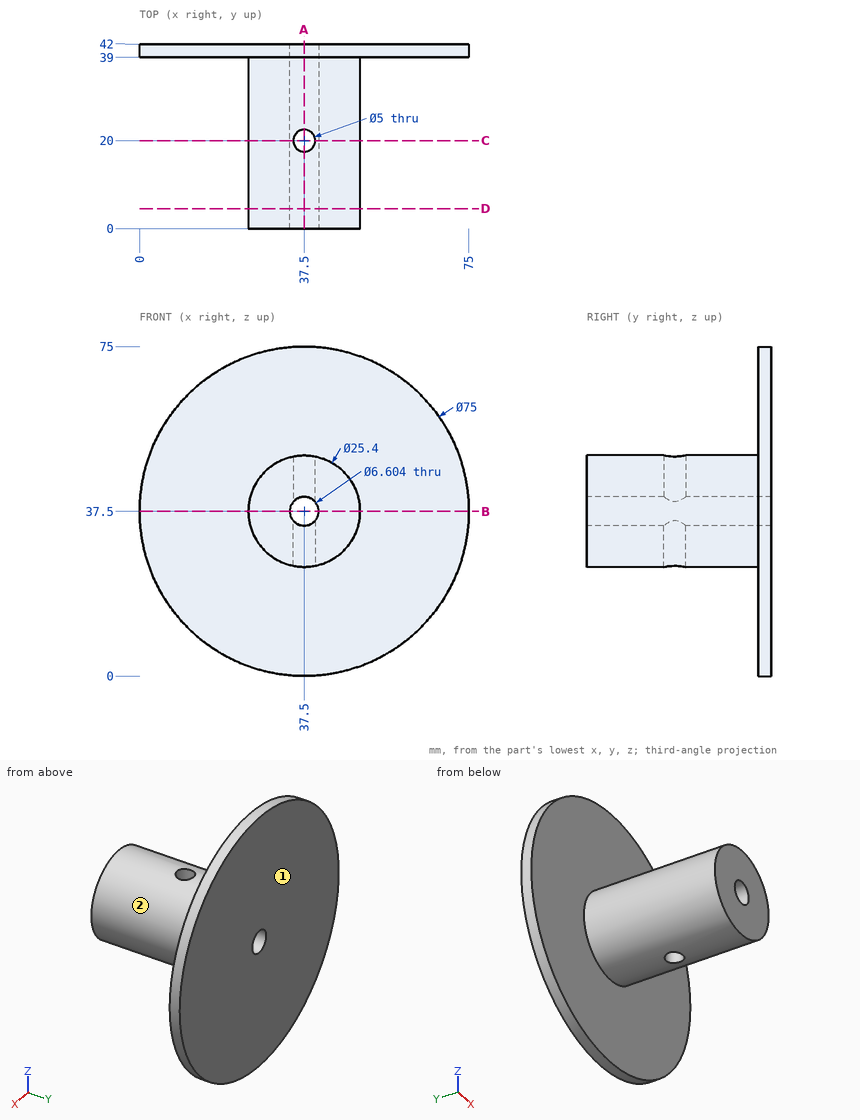
The figure shows three views and two pictorial views of one solid part (mm, origin at its lowest corner). Answer the questions. A direction names the side the tool comes from. Round coordinates to 2 decimals unless told otherwise and drop trailing zeros. Order: outer loops, then holes, each group sorted by start corner. A loop starts at its lowest first (then second) coordinate and runs counter-clockwise, first axis right, second up. Notation, with made-up numbers: (75, 75.5) -> (99, 75.5) arc R34 ccw to (99, 106.5) -> close; hole circle Ø2 at (22.5, -15). An arc over 180 degrees is marked (long way). Put each result on its own line as item: value.
Q1. Section D-D, the plane y = 4.5 is taken. Write down the section's boundary in (x, z), and give its area (3 significant figures).
Results list:
outline: circle Ø25.4 at (37.5, 37.5); hole circle Ø6.6 at (37.5, 37.5)
area: 472 mm^2
Q2. Section C-C, the plane y = 20 is taken. Write down the section's boundary in (x, z), and give its area (3 significant figures).
Results list:
outline: (35, 25.05) -> (35, 35.34) arc R3.3 cw to (35, 39.66) -> (35, 49.95) arc R12.7 ccw to start; (40, 25.05) arc R12.7 ccw to (40, 49.95) -> (40, 39.66) arc R3.3 cw to (40, 35.34) -> close
area: 376 mm^2
Q3. Section A-A, the plane x = 37.5 is taken. Write down the section's boundary in (y, z).
Results list:
outline: (0, 24.8) -> (17.5, 24.8) -> (17.5, 34.2) -> (0, 34.2) -> close; (0, 40.8) -> (17.5, 40.8) -> (17.5, 50.2) -> (0, 50.2) -> close; (22.5, 24.8) -> (39, 24.8) -> (39, 0) -> (42, 0) -> (42, 34.2) -> (22.5, 34.2) -> close; (22.5, 40.8) -> (42, 40.8) -> (42, 75) -> (39, 75) -> (39, 50.2) -> (22.5, 50.2) -> close
Q4. Which of the six approach directions +Z, -Z, +X, -X, +Y, -Y give full straight-line access (tool end or side, diameter ignored) to the marked faces 1 and 2?
Results list:
face 1: +Z, -Z, +X, -X, +Y
face 2: -Y
Q5. Consider line 1 along Z through (x, y) = (37.5, 24.5); line 2 along X through (y, z) = (2.5, 40.5). Determine where each line is inside the solid, lowest interval first.
Results list:
line 1: 24.8 to 34.2, 40.8 to 50.2
line 2: 25.16 to 36.12, 38.88 to 49.84
Q6. Section B-B, the plane z = 37.5 is taken. Write down the section's boundary in (x, y).
Results list:
outline: (0, 39) -> (24.8, 39) -> (24.8, 0) -> (34.2, 0) -> (34.2, 42) -> (0, 42) -> close; (40.8, 0) -> (50.2, 0) -> (50.2, 39) -> (75, 39) -> (75, 42) -> (40.8, 42) -> close
Q7. Each of these flat-tipped pins is pushed along its axis until it touches: P1, Ø6, axis at x = 37.5, y = 20, coming from the -Z side; P2, Ø6, axis at x = 66, z = 58.5, coming from the -Y side; P3, Ø6, axis at x = 45, y = 32, coming from the -Z side. Where does it stop, or does it pass through?
Results list:
P1: z = 24.8
P2: y = 39
P3: z = 25.62
